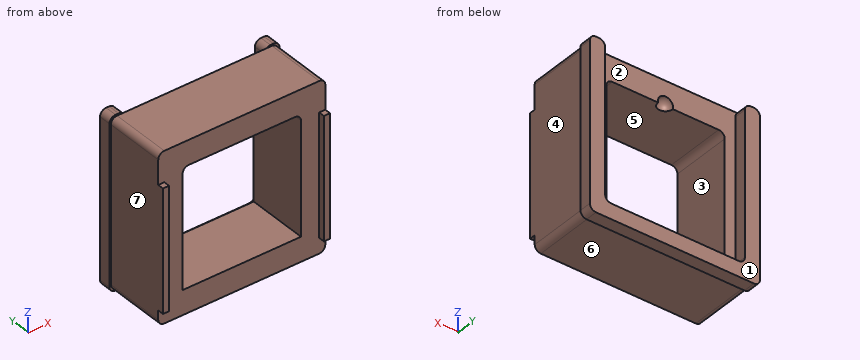
```python
from build123d import *
from build123d.topology import SkipClean

# Parameters (mm, degrees)
BOSS_EXTRUDE1_DEPTH = 2
SKETCH3_W           = 27.5
SKETCH3_H           = 27.5
SKETCH3_W_2         = 19.5
SKETCH3_H_2         = 19.5
BOSS_EXTRUDE2_DEPTH = 10
SKETCH4_W           = 1
SKETCH4_H           = 20
BOSS_EXTRUDE3_DEPTH = 1
FILLET2_R           = 1


with BuildPart() as part:
    # Sketch1 → Boss-Extrude1 (new body)
    with BuildSketch(Plane(origin=(0, 0, 0), x_dir=(1, 0, 0), z_dir=(0, 1, 0))):
        Polygon((-14, 14), (-14, -14), (-11.5, -14), (-11.5, 11.5), (11.5, 11.5), (11.5, -14), (14, -14), (14, 14), align=None)
    extrude(amount=BOSS_EXTRUDE1_DEPTH)

    # Sketch3 → Boss-Extrude2 (add)
    with BuildSketch(Plane.XZ):
        Rectangle(SKETCH3_W, SKETCH3_H)
        Rectangle(SKETCH3_W_2, SKETCH3_H_2, mode=Mode.SUBTRACT)
    extrude(amount=BOSS_EXTRUDE2_DEPTH)

    # Sketch4 → Boss-Extrude3 (add)
    with BuildSketch(Plane.XZ.offset(10)):
        with Locations((-13.25, -1.25)):
            Rectangle(SKETCH4_W, SKETCH4_H)
        with Locations((13.25, -1.25)):
            Rectangle(SKETCH4_W, SKETCH4_H)
    extrude(amount=BOSS_EXTRUDE3_DEPTH)

    # Sketch5 → Cut-Revolve4 (revolve, cut)
    with SkipClean():  # the faces are left unmerged after this step: merging them gives an invalid solid
        with BuildSketch(Plane(origin=(0, 0, 0), x_dir=(0, 0, -1), z_dir=(1, 0, 0))):
            with BuildLine():
                ThreePointArc((-8.75, 0), (-10, 1.25), (-11.25, 0))
                Line((-11.25, 0), (-8.75, 0))
            make_face()
            with BuildLine():
                Line((-8.75, 0), (-11.25, 0))
                ThreePointArc((-11.25, 0), (-10, -1.25), (-8.75, 0))
            make_face()
        revolve(axis=Axis((0, 0, 1000), (0, 0, -1)), mode=Mode.SUBTRACT)
    add(part.part.scale(1), mode=Mode.REPLACE)  # the faces are merged on a copy

    # Fillet2
    # the kernel refuses this fillet: 1 mm, written as the material it adds along each edge
    with BuildSketch(Plane(origin=(11.5, -2.5, -11.5), x_dir=(0, 0, 1), z_dir=(0, 1, 0))) as fillet2_piece_1:
        with BuildLine():
            CenterArc((FILLET2_R, -FILLET2_R), FILLET2_R, 90, 90)
            Line((0, -FILLET2_R), (0, 0))
            Line((0, 0), (FILLET2_R, 0))
        make_face()
    extrude(amount=4.5)
    with BuildSketch(Plane(origin=(-11.5, -2.5, -11.5), x_dir=(0, 0, 1), z_dir=(0, 1, 0))) as fillet2_piece_2:
        with BuildLine():
            CenterArc((FILLET2_R, FILLET2_R), FILLET2_R, 180, 90)
            Line((0, FILLET2_R), (0, 0))
            Line((0, 0), (FILLET2_R, 0))
        make_face()
    extrude(amount=4.5)
    with BuildSketch(Plane(origin=(-9.75, 0, 9.75), x_dir=(0, 0, -1), z_dir=(0, -1, 0))) as fillet2_piece_3:
        with BuildLine():
            CenterArc((FILLET2_R, FILLET2_R), FILLET2_R, 180, 90)
            Line((0, FILLET2_R), (0, 0))
            Line((0, 0), (FILLET2_R, 0))
        make_face()
    extrude(amount=10)
    with BuildSketch(Plane(origin=(9.75, 0, 9.75), x_dir=(0, 0, -1), z_dir=(0, -1, 0))) as fillet2_piece_4:
        with BuildLine():
            CenterArc((FILLET2_R, -FILLET2_R), FILLET2_R, 90, 90)
            Line((0, -FILLET2_R), (0, 0))
            Line((0, 0), (FILLET2_R, 0))
        make_face()
    extrude(amount=10)
    # the kernel refuses this fillet: 1 mm, written as the material it takes off along each edge
    with BuildSketch(Plane(origin=(-11.5, 0, 14), x_dir=(-1, 0, 0), z_dir=(0, 1, 0))) as fillet2_2_piece_1:
        with BuildLine():
            CenterArc((FILLET2_R, -FILLET2_R), FILLET2_R, 90, 90)
            Line((0, -FILLET2_R), (0, 0))
            Line((0, 0), (FILLET2_R, 0))
        make_face()
    extrude(amount=4.5, mode=Mode.SUBTRACT)
    with BuildSketch(Plane(origin=(-14, -2.5, 14), x_dir=(0, 0, -1), z_dir=(0, 1, 0))) as fillet2_2_piece_2:
        with BuildLine():
            CenterArc((FILLET2_R, -FILLET2_R), FILLET2_R, 90, 90)
            Line((0, -FILLET2_R), (0, 0))
            Line((0, 0), (FILLET2_R, 0))
        make_face()
    extrude(amount=7, mode=Mode.SUBTRACT)
    with BuildSketch(Plane(origin=(-14, -2.5, -14), x_dir=(0, 0, 1), z_dir=(0, 1, 0)), Plane(origin=(14, -2.5, -14), x_dir=(-1, 0, 0), z_dir=(0, 1, 0)), Plane(origin=(14, -2.5, 14), x_dir=(0, 0, -1), z_dir=(0, 1, 0))) as fillet2_2_piece_3:
        with BuildLine():
            CenterArc((FILLET2_R, FILLET2_R), FILLET2_R, 180, 90)
            Line((0, FILLET2_R), (0, 0))
            Line((0, 0), (FILLET2_R, 0))
        make_face()
    extrude(amount=7, mode=Mode.SUBTRACT)
    with BuildSketch(Plane(origin=(11.5, 0, 14), x_dir=(1, 0, 0), z_dir=(0, 1, 0))) as fillet2_2_piece_4:
        with BuildLine():
            CenterArc((FILLET2_R, FILLET2_R), FILLET2_R, 180, 90)
            Line((0, FILLET2_R), (0, 0))
            Line((0, 0), (FILLET2_R, 0))
        make_face()
    extrude(amount=4.5, mode=Mode.SUBTRACT)
    with BuildSketch(Plane(origin=(13.75, 0, 13.75), x_dir=(-1, 0, 0), z_dir=(0, -1, 0)), Plane(origin=(-13.75, 0, -13.75), x_dir=(1, 0, 0), z_dir=(0, -1, 0)), Plane(origin=(13.75, 0, -13.75), x_dir=(0, 0, 1), z_dir=(0, -1, 0))) as fillet2_2_piece_5:
        with BuildLine():
            CenterArc((FILLET2_R, FILLET2_R), FILLET2_R, 180, 90)
            Line((0, FILLET2_R), (0, 0))
            Line((0, 0), (FILLET2_R, 0))
        make_face()
    extrude(amount=12.5, mode=Mode.SUBTRACT)
    with BuildSketch(Plane(origin=(-13.75, 0, 13.75), x_dir=(1, 0, 0), z_dir=(0, -1, 0))) as fillet2_2_piece_6:
        with BuildLine():
            CenterArc((FILLET2_R, -FILLET2_R), FILLET2_R, 90, 90)
            Line((0, -FILLET2_R), (0, 0))
            Line((0, 0), (FILLET2_R, 0))
        make_face()
    extrude(amount=12.5, mode=Mode.SUBTRACT)


solid = part.part
```
Check sheet for the modelled part. Datum: model origin and axes. Units: mm. Face numbers are marked on the shaded views. A direction names the side the tool comes from. Round coordinates to 2 decimals unless told otherwise and drop trailing zeros. Order: outer loops, then holes, each group sorted by start corner. A loop starts at its lowest first (then second) coordinate and runs counter-clockwise, first axis right, second up. Notation, with made-up numbers: M -35,61.5 L -20,61.5 A35 cw -20,95.5 Z; hole C 15.25,49 d7. An arc over 180 degrees is marked long. Answer in a Markdown table with one row per item.
(1) Gauge pin test, flat ends, axial feed: pin 1 (0.8 mm diameter, centred on x = -13, y = -10.5, fed in from -Z); pin 2 (1 mm diameter, centred on x = -4, y = 1, fed in from +Z); pin 3 (3 mm diameter, centred on x = -1, y = -6.5, fed in from +Z). Record the tip position at first contact, or that the pin passes through.
Findings:
| item | result |
|---|---|
| pin 1 | stops at z = -11.25 |
| pin 2 | stops at z = -11.5 |
| pin 3 | stops at z = 13.75 |
(2) Draft check along Z on the marked faces 5, 6 and 7. Enter one of: +Z half, -Z half, draft (parallel to the pull), parting line (faces both ways), or undercut.
Findings:
| item | result |
|---|---|
| face 5 | undercut |
| face 6 | -Z half |
| face 7 | draft |
(3) Section check C-C on z = 7.5. Record the boundary of the cut face in (x, y).
Findings:
| item | result |
|---|---|
| outline | M -14,0 L -13.75,0 L -13.75,-11 L -12.75,-11 L -12.75,-10 L -9.75,-10 L -9.75,0 L -11.5,0 L -11.5,2 L -14,2 Z; M 9.75,-10 L 12.75,-10 L 12.75,-11 L 13.75,-11 L 13.75,0 L 14,0 L 14,2 L 11.5,2 L 11.5,0 L 9.75,0 Z |
(4) Section check B-B on y = -5.25. Record the boundary of the cut face in (x, z).
Findings:
| item | result |
|---|---|
| outline | M -13.75,-12.75 A1 ccw -12.75,-13.75 L 12.75,-13.75 A1 ccw 13.75,-12.75 L 13.75,12.75 A1 ccw 12.75,13.75 L -12.75,13.75 A1 ccw -13.75,12.75 Z; hole M -9.75,-9.75 L 9.75,-9.75 L 9.75,8.75 A1 ccw 8.75,9.75 L -8.75,9.75 A1 ccw -9.75,8.75 Z |
(5) Material ranges on line 1 along Z through (x, y) = (6.75, -7); line 2 along X through (y, z) = (1.5, 9.5), recorded low to high. Write a range as from..to.
Findings:
| item | result |
|---|---|
| line 1 | z = -13.75..-9.75, 9.75..13.75 |
| line 2 | x = -14..-11.5, 11.5..14 |
(6) Section check A-A on x = -4.5. Record the boundary of the cut face in (y, z).
Findings:
| item | result |
|---|---|
| outline | M -10,-13.75 L 0,-13.75 L 0,-14 L 2,-14 L 2,-11.5 L 0,-11.5 L 0,-9.75 L -10,-9.75 Z; M -10,9.75 L 0,9.75 L 0,13.75 L -10,13.75 Z |
(7) Section check D-D on y = 0.5. Record the boundary of the cut face in (x, z), plus the area to 3 significant figures.
Findings:
| item | result |
|---|---|
| outline | M -14,-13 A1 ccw -13,-14 L 13,-14 A1 ccw 14,-13 L 14,13 A1 ccw 13,14 L 12.5,14 A1 ccw 11.5,13 L 11.5,-10.5 A1 cw 10.5,-11.5 L -10.5,-11.5 A1 cw -11.5,-10.5 L -11.5,13 A1 ccw -12.5,14 L -13,14 A1 ccw -14,13 Z |
| area | 197 mm^2 |
(8) Set-up check for the marked faces 1, 2, 3 and 4: record each of +Z, -Z, +X, -X, +Y, -Y from which the full face is reachable in a straight line by a thin tool's end or side.
Findings:
| item | result |
|---|---|
| face 1 | +Z, -Z, +X, -X, +Y |
| face 2 | +Z, +Y |
| face 3 | +Y, -Y |
| face 4 | +Z, -Z, +X, -Y |
